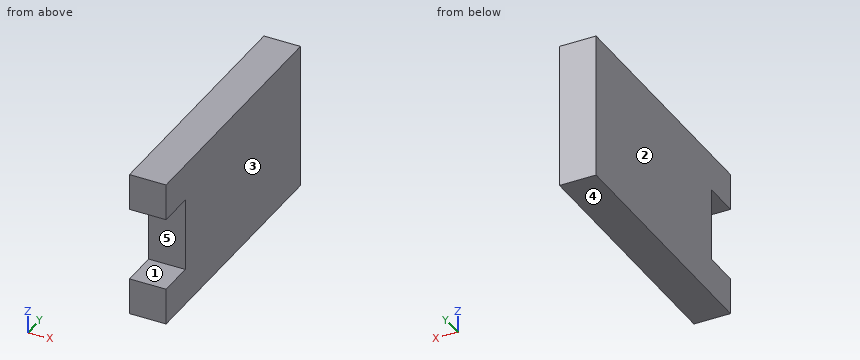
from build123d import *

# Parameters (mm, degrees)
SKETCH1_W           = 6.35
SKETCH1_H           = 6.35
BOSS_EXTRUDE1_DEPTH = 6.35


with BuildPart() as part:
    # Sketch1 → Boss-Extrude1 (new body)
    with BuildSketch(Plane(origin=(0, 0, 0), x_dir=(0, 0, -1), z_dir=(1, 0, 0))):
        Polygon((-12.7, -12.7), (-12.7, -19.05), (-6.35, -19.05), (6.35, -19.05), (12.7, -19.05), (12.7, 19.05), (-12.7, 19.05), align=None)
        with Locations((-9.525, -22.225)):
            Rectangle(SKETCH1_W, SKETCH1_H)
        with Locations((9.525, -22.225)):
            Rectangle(SKETCH1_W, SKETCH1_H)
    extrude(amount=BOSS_EXTRUDE1_DEPTH)


solid = part.part
For this review, take the finished solid that the model builds, in its own axes (mm). Face numbers are marked on the shaded views. A direction names the side the tool comes from. Round coordinates to 2 decimals unless told otherwise and drop trailing zeros. Write each loop counter-clockwise with the first axis right and the second up, starting at its lowest first coordinate (ties: lowest second). Pieces come first, ordered by that corner, then holes. Notation, with made-up numbers: M 67,-8 L 112,-8 A14 cw 112,-1 Z; hole C 22.5,-40 d3. An arc over 180 degrees is marked long. Write item = value, one per line. Start each with the question number.
(1) We need section C-C (z = 2.25). Give the boundary of the cut face in (x, y), then the cut area to 3 significant figures.
(2) We need section B-B (x = 5). Give the boundary of the cut face in (y, z).
(3) For line 1 along Y through (x, z) = (1.25, 0.5), list the stretches that pass through material, from the lowest coordinate up.
(4) The part is to be moulded in two halves that separate along Z. For the marked faces 3, 4 and 5, say which applies: +Z half, -Z half, draft (parallel to the pull), parting line (faces both ways), or undercut.
(5) Clearance check with a flat-ended pin moving along its axis: pin 1 Ø1 at (y, z) = (-0.5, 8.5) entering from -X. State where the tip first meets the part, or that it passes through.
(6) We need section A-A (y = -19.5). Give the boundary of the cut face in (x, z).
(7) For the marked faces 1 and 2, list the 3-axis set-ups (+Z, -Z, +X, -X, +Y, -Y) from which the entire face can be reached by the end or side of a thin tool; tool diameter is ignored.
Results found:
q1.outline = M 0,-19.05 L 6.35,-19.05 L 6.35,19.05 L 0,19.05 Z
q1.area = 242 mm²
q2.outline = M -25.4,-12.7 L 19.05,-12.7 L 19.05,12.7 L -25.4,12.7 L -25.4,6.35 L -19.05,6.35 L -19.05,-6.35 L -25.4,-6.35 Z
q3.line_1 = -19.05 to 19.05
q4.face_3 = draft
q4.face_4 = -Z half
q4.face_5 = undercut
q5.pin_1 = 0
q6.outline = M 0,-12.7 L 6.35,-12.7 L 6.35,-6.35 L 0,-6.35 Z; M 0,6.35 L 6.35,6.35 L 6.35,12.7 L 0,12.7 Z
q7.face_1 = +X, -X, -Y
q7.face_2 = +Z, -Z, -X, +Y, -Y
